from build123d import *

# Parameters (mm, degrees)
SKETCH1_R           = 10
BOSS_EXTRUDE1_DEPTH = 35
SKETCH2_R           = 15
BOSS_EXTRUDE2_DEPTH = 5
CHAMFER1_SIZE       = 1


with BuildPart() as part:
    # Sketch1 → Boss-Extrude1 (new body)
    with BuildSketch(Plane.XY):
        Circle(SKETCH1_R)
    extrude(amount=-BOSS_EXTRUDE1_DEPTH)

    # Sketch2 → Boss-Extrude2 (add)
    with BuildSketch(Plane.XY):
        Circle(SKETCH2_R)
    extrude(amount=BOSS_EXTRUDE2_DEPTH)

    # Chamfer1
    chamfer1_edges = [part.edges().sort_by_distance(p)[0] for p in [
        (-10, 0, -35),
    ]]
    chamfer(chamfer1_edges, length=CHAMFER1_SIZE)


solid = part.part
Here's how the part is built. I have some questions about the finished solid (model axes, mm). A direction names the side the tool comes from. Round coordinates to 2 decimals unless told otherwise and drop trailing zeros. Loops run counter-clockwise (first coordinate to the right, second up) from the corner with the lowest first, then second, coordinate; pieces in that order, holes last.
1. If we section it at C-C on z = -11: Write out the boundary of the cut face in (x, y).
Answer list:
outline: circle Ø20 at (0, 0)
2. We'd pull the mould along Y, two halves only. Please class faces 1 (the face through (0, 0, -35)), 2 (the face through (-2.17, -9.76, -16.76)): +Y half, -Y half, draft (parallel to the pull), parting line (faces both ways), or undercut.
Answer list:
face 1: draft
face 2: parting line
3. Which directions (+Z, -Z, +X, -X, +Y, -Y) give clear straight access to the entire face, cutting with the end or side of a thin tool? Please do faces 3 (the face through (-14.985, 0.66, 2.465)), 4 (the face through (3, -10, 0)).
Answer list:
face 3: +Z, -Z
face 4: -Z
4. If we section it at A-A on x = 0: Write out the boundary of the cut face in (y, z).
Answer list:
outline: (-15, 0) - (-10, 0) - (-10, -34) - (-9, -35) - (9, -35) - (10, -34) - (10, 0) - (15, 0) - (15, 5) - (-15, 5) - close
5. If we section it at D-D on y = -10.5: Write out the boundary of the cut face in (x, z), plus the area to 3 significant figures.
Answer list:
outline: (-10.71, 0) - (10.71, 0) - (10.71, 5) - (-10.71, 5) - close
area: 107 mm2
6. For P1, Ø8, axis at x = -6.5, z = -8.5, coming from the -Y side; P2, Ø6, axis at y = -7, z = -2.5, coming from the +X side; P3, Ø8, axis at x = -0.5, z = -27, coming from the +Y side, each with a flat end and sliding along its axis, tell me the tip position at first contact or that it passes through.
Answer list:
P1: stops at y = -9.68
P2: stops at x = 14.02
P3: stops at y = 10
7. If I drill on line 1 along Z through (x, y) = (10.25, 7.25); line 2 along X through (y, z) = (2.5, -24); line 3 along X through (y, z) = (-8, -17), over which ranges is the centre line in solid material (lowest first)?
Answer list:
line 1: z = 0 to 5
line 2: x = -9.68 to 9.68
line 3: x = -6 to 6
